Verification items for the finished model (mm, model axes). A direction names the side the tool comes from. Give positions to 0.01 mm unless a question says otherwise; leave off trailing zeros. Loops run counter-clockwise (first coordinate to the right, second up) from the corner with the lowest first, then second, coordinate; pieces in that order, holes last. Notation, with made-up numbers: M -40,-9.75 L -9,-9.75 A10 ccw -9,3.25 Z; hole C -31.5,78 d10. An arc over 180 degrees is marked long. Answer in a Markdown table with one row per item.
Autodesk Inventor part; units mm, degrees
ref_plane "YZ Plane" through (0, 0, 0) normal (1, 0, 0) x (0, 1, 0)
ref_plane "XZ Plane" through (0, 0, 0) normal (0, 1, 0) x (-1, 0, 0)
ref_plane "XY Plane" through (0, 0, 0) normal (0, 0, 1) x (1, 0, 0)
sketch "Sketch1" plane through (0, 0, 0) normal (0, 0, 1) x (1, 0, 0)
  line L0 (0, 0) -> (0, 47.4625)
  line L1 (0, 47.4625) -> (27.4025, 94.925)
  line L2 (27.4025, 94.925) -> (82.2075, 94.925)
  line L3 (82.2075, 94.925) -> (109.61, 47.4625)
  line L4 (109.61, 47.4625) -> (109.61, 0)
  line L5 (109.61, 0) -> (0, 0)
  dimension "d2" = 54.805
  dimension "d3" = 120
  dimension "d4" = 120
  dimension "d5" = 47.4625
  dimension "d6" = 47.4625
extrude "Extrusion1" add sketch "Sketch1" along normal blind 6
sketch "Sketch2" plane through (0, 0, 6) normal (0, 0, 1) x (1, 0, 0)
  line L0 (0, 47.4625) -> (0, 0)
  line L1 (0, 0) -> (109.61, 0)
  line L2 (109.61, 0) -> (109.61, 47.4625)
  line L3 (109.61, 47.4625) -> (82.2075, 94.925)
  line L4 (82.2075, 94.925) -> (27.4025, 94.925)
  line L5 (27.4025, 94.925) -> (0, 47.4625)
  circle A0 centre (5, 28) radius 1.01
  circle A1 centre (5, 10) radius 1.01
  circle A2 centre (104.61, 28) radius 1.01
  circle A3 centre (104.61, 10) radius 1.01
  circle A4 centre (44.6125, 84.925) radius 1.6
  circle A5 centre (64.9975, 84.925) radius 1.6
  line L6 (7, 30.695) -> (16.57, 30.695)
  line L7 (16.57, 30.695) -> (16.57, 7.305)
  line L8 (16.57, 7.305) -> (7, 7.305)
  line L9 (7, 7.305) -> (7, 30.695)
  line L10 (93.04, 30.695) -> (102.61, 30.695)
  line L11 (102.61, 30.695) -> (102.61, 7.305)
  line L12 (102.61, 7.305) -> (93.04, 7.305)
  line L13 (93.04, 7.305) -> (93.04, 30.695)
  line L14 (82.2075, 94.925) -> (27.4025, 94.925) construction
  line L15 (54.805, 94.925) -> (54.805, 91.0637) construction
  line L16 (5, 28) -> (5, 10) construction
  line L17 (5, 19) -> (11.5154, 19) construction
  dimension "d10" = 2.02
  dimension "d11" = 3.2
  dimension "d12" = 5
  dimension "d13" = 5
  dimension "d14" = 18
  dimension "d15" = 10
  dimension "d16" = 23.39
  dimension "d17" = 9.57
  dimension "d19" = 2
  dimension "d20" = 2
  dimension "d21" = 20.385
  dimension "d22" = 10
  dimension "d23" = 3.8614
extrude "Extrusion2" cut sketch "Sketch2" against normal through all contours A0 | A1 | A2 | A3 | A4 | A5 | L6 L7 L8 L9 | L10 L11 L12 L13
sketch "Sketch3" plane through (0, 0, 6) normal (0, 0, 1) x (1, 0, 0)
  line L0 (7, 7.305) -> (7, 30.695)
  line L1 (7, 30.695) -> (16.57, 30.695)
  line L2 (16.57, 30.695) -> (16.57, 7.305)
  line L3 (16.57, 7.305) -> (7, 7.305)
  circle A0 centre (44.6125, 84.925) radius 1.6
  circle A1 centre (104.61, 28) radius 1.01
  circle A2 centre (5, 28) radius 1.01
  circle A3 centre (5, 10) radius 1.01
  circle A4 centre (104.61, 10) radius 1.01
  circle A5 centre (64.9975, 84.925) radius 1.6
  line L4 (93.04, 7.305) -> (93.04, 30.695)
  line L5 (93.04, 30.695) -> (102.61, 30.695)
  line L6 (102.61, 30.695) -> (102.61, 7.305)
  line L7 (102.61, 7.305) -> (93.04, 7.305)
  line L8 (0, 47.4625) -> (0, 0)
  line L9 (0, 0) -> (109.61, 0)
  line L10 (109.61, 0) -> (109.61, 47.4625)
  line L11 (109.61, 47.4625) -> (82.2075, 94.925)
  line L12 (82.2075, 94.925) -> (27.4025, 94.925)
  line L13 (27.4025, 94.925) -> (0, 47.4625)
  line L14 (82.2075, 94.925) -> (109.61, 47.4625)
  line L15 (109.61, 47.4625) -> (82.2075, 0)
  line L16 (82.2075, 0) -> (27.4025, 0)
  line L17 (27.4025, 0) -> (0, 47.4625)
  line L18 (0, 47.4625) -> (27.4025, 94.925)
  line L19 (27.4025, 94.925) -> (82.2075, 94.925)
  circle A6 centre (33.055, 77.3404) radius 1.55
  circle A7 centre (39.805, 81.2375) radius 1.55
  circle A8 centre (69.805, 81.2375) radius 1.55
  circle A9 centre (18.055, 51.3596) radius 1.55
  circle A10 centre (18.055, 43.5654) radius 1.55
  circle A11 centre (33.055, 17.5846) radius 1.55
  circle A12 centre (39.805, 13.6875) radius 1.55
  circle A13 centre (69.805, 13.6875) radius 1.55
  circle A14 centre (76.555, 17.5846) radius 1.55
  circle A15 centre (91.555, 43.5654) radius 1.55
  circle A16 centre (91.555, 51.3596) radius 1.55
  line L20 (74.305, 81.2375) -> (93.805, 47.4625) construction
  line L21 (93.805, 47.4625) -> (74.305, 13.6875) construction
  line L22 (74.305, 13.6875) -> (35.305, 13.6875) construction
  line L23 (35.305, 13.6875) -> (15.805, 47.4625) construction
  line L24 (15.805, 47.4625) -> (35.305, 81.2375) construction
  line L25 (35.305, 81.2375) -> (74.305, 81.2375) construction
  circle A17 centre (76.555, 77.3404) radius 1.55
  point P0 (54.805, 47.4625)
  point P1 (54.805, 47.4625)
  dimension "d26" = 3.1
  dimension "d27" = 39
  dimension "d28" = 4.5
  dimension "d29" = 4.5
  dimension "d30" = 4.5
  dimension "d31" = 4.5
  dimension "d32" = 4.5
  dimension "d33" = 4.5
  dimension "d34" = 4.5
  dimension "d35" = 4.5
  dimension "d36" = 4.5
  dimension "d37" = 4.5
  dimension "d40" = 59.7557
extrude "Extrusion3" cut sketch "Sketch3" against normal through all contours A6 | A7 | A8 | A9 | A10 | A11 | A12 | A13 | A14 | A15 | A16 | A17
fillet "Fillet1" radius 4 6 edges at (109.61, 0, 3) (109.61, 47.4625, 3) (82.2075, 94.925, 3) (27.4025, 94.925, 3) (0, 47.4625, 3) (0, 0, 3)
equation "\"d4\" = d3"
equation "\"d6\" = d5"
equation "\"d13\" = d12"
equation "\"d20\" = d19"
equation "\"d29\" = d28"
equation "\"d30\" = d28"
equation "\"d31\" = d29"
equation "\"d32\" = d28"
equation "\"d33\" = d28"
equation "\"d34\" = d28"
equation "\"d35\" = d28"
equation "\"d36\" = d28"
equation "\"d37\" = d30"
properties part number "megapr"
Item 1: Go/stop test with flat-tipped pins: pin 1 (1.6 mm diameter, centred on x = 5, y = 28, fed in from +Z); pin 2 (1 mm diameter, centred on y = 66, z = 0.5, fed in from -X); pin 3 (2 mm diameter, centred on y = 52.5, z = 4, fed in from -X); pin 4 (3 mm diameter, centred on x = 9.5, z = 3.5, fed in from +Y). Record where each tip stops, or that it passes through.
Reported:
| item | result |
|---|---|
| pin 1 | passes through |
| pin 2 | stops at x = 10.41 |
| pin 3 | stops at x = 2.33 |
| pin 4 | stops at y = 66.52 |
Item 2: Scan lines: L1, parallel to X at y = 12, z = 5.85; L2, parallel to Y at x = 12, z = 4.5 (3 decimals); L3, parallel to X at y = 52.5, z = 2.1. Record each from-to range of solid material in increasing order. Write a range as [from, to].
Reported:
| item | result |
|---|---|
| L1 | x = [0, 7], [16.57, 93.04], [102.61, 109.61] |
| L2 | y = [0, 7.305], [30.695, 68.247] |
| L3 | x = [2.91, 17.01], [19.1, 90.51], [92.6, 106.7] |
Item 3: Sectioned sample at A-A (x = 65). Record the cut outline in (y, z) (3 decimals).
Reported:
| item | result |
|---|---|
| outline | M 0,0 L 83.325,0 L 83.325,6 L 0,6 Z; M 86.525,0 L 94.925,0 L 94.925,6 L 86.525,6 Z |
Item 4: Sectioned sample at B-B (z = 4.7). State how many separate pieces and enclosed holes the cut face has, and give its area (3 significant figures).
Reported:
| item | result |
|---|---|
| separate pieces | 1 |
| enclosed holes | 20 |
| area | 8,530 mm^2 |
Item 5: Tool access check on faces 1 (the cylindrical face through (108.407, 1.141, 3.042)), 2 (the flat face through (16.57, 19, 3)). Record the directions out of +Z, -Z, +X, -X, +Y, -Y that give a thin tool (end or side, any length) a straight path to the whole face; none if there is none.
Reported:
| item | result |
|---|---|
| face 1 | +Z, -Z, +X, -Y |
| face 2 | +Z, -Z |
Item 6: Sectioned sample at C-C (y = 73). Record the cut outline in (x, z), and give its area (3 significant figures).
Reported:
| item | result |
|---|---|
| outline | M 14.74,0 L 94.87,0 L 94.87,6 L 14.74,6 Z |
| area | 481 mm^2 |
Item 7: Release check for a two-part mould opening along X. For faces 3 (the flat face through (7, 19, 3)), 4 (the flat face through (96.04, 70.97, 2.96)), 5 (the flat face through (13.212, 70.346, 2.958)) record: released by +X, released by -X, zero draft, split by the parting line, or undercut.
Reported:
| item | result |
|---|---|
| face 3 | undercut |
| face 4 | released by +X |
| face 5 | released by -X |
